from build123d import *

# Parameters (mm, degrees)
F0_W     = 11.4046361996
F0_H     = 20.0534798205
F1_DEPTH = 12.7
F3_DEPTH = 4.17264
F5_R     = 3.1549889686
F6_DEPTH = 25.4
F7_W     = 10.0605683401
F7_H     = 14.2366550863
F8_DEPTH = 7.95975


with BuildPart() as f1:
    # F0 (on Front) → F1 (new body, symmetric)
    with BuildSketch(Plane.XZ):
        Polygon((-13.2875442505, 21.1651604623), (-17.2738078982, 0), (-13.2875442505, 0), (-1.8829080509, 0), (0, 0), (0, 21.1651604623), align=None)
        with Locations((-7.5852261507, -10.0267399102)):
            Rectangle(F0_W, F0_H)
        Polygon((13.2875442505, 21.1651604623), (0, 21.1651604623), (0, 0), (1.8829080509, 0), (13.2875442505, 0), (17.2738078982, 0), align=None)
        with Locations((7.5852261507, -10.0267399102)):
            Rectangle(F0_W, F0_H)
    extrude(amount=F1_DEPTH, both=True)

    # F2 (on face) → F3 (join)
    with BuildSketch(Plane(origin=(-16.6820575494, 0, 3.1419123751), x_dir=(0, -1, 0), z_dir=(-0.982722195, 0, 0.1850867027))):
        with BuildLine():
            Line((-13.796438463, 1.4029195299), (0, 2.9041063972))
            ThreePointArc((0, 2.9041063972), (5.3533335924, 7.9779976513), (0, 13.0518889055))
            Line((0, 13.0518889055), (-7.7627915889, 8.660916239))
            Line((-7.7627915889, 8.660916239), (-19.0092052332, 5.8628071696))
            ThreePointArc((-19.0092052332, 5.8628071696), (-18.616808085, 4.3270320221), (-19.026460126, 2.7957691345))
            Line((-19.026460126, 2.7957691345), (-13.796438463, 1.4029195299))
        make_face()
        with BuildLine():
            ThreePointArc((-23.0272375047, 1.4844691614), (-20.7737198496, 1.3678224494), (-19.026460126, 2.7957691345))
            ThreePointArc((-19.026460126, 2.7957691345), (-18.616808085, 4.3270320221), (-19.0092052332, 5.8628071696))
            ThreePointArc((-19.0092052332, 5.8628071696), (-21.0317417116, 7.3939934823), (-23.5248878598, 6.9255838171))
            Line((-23.5248878598, 6.9255838171), (-23.5248878598, 5.4076067172))
            ThreePointArc((-23.5248878598, 5.4076067172), (-19.7584909862, 4.1445688112), (-23.5248878598, 2.8815309051))
            Line((-23.5248878598, 2.8815309051), (-23.0272375047, 1.4844691614))
        make_face()
    extrude(amount=F3_DEPTH)

    # F4: F1 across plane


with BuildPart() as f1_1:
    add(f1.part)
    add(f1.part.mirror(Plane.YZ))

    # F5 (on Top) → F6 (join)
    with BuildSketch(Plane.XY):
        Circle(F5_R)
    extrude(amount=F6_DEPTH)

    # F7 (on Front) → F8 (join)
    with BuildSketch(Plane.XZ):
        with Locations((5.0302841701, 30.1817078143)):
            Rectangle(F7_W, F7_H)
        with Locations((-5.0302841701, 30.1817078143)):
            Rectangle(F7_W, F7_H)
    extrude(amount=-F8_DEPTH)


solid = f1_1.part
Geometry check sheet. Reference: the model listing, model coordinates, mm. A direction names the side the tool comes from. Round coordinates to 2 decimals unless told otherwise and drop trailing zeros. Write each loop counter-clockwise with the first axis right and the second up, starting at its lowest first coordinate (ties: lowest second). Pieces come first, ordered by that corner, then holes. Notation, with made-up numbers: (15, 65) -> (29, 65) arc R18 ccw to (29, 95) -> close; hole circle Ø6 at (65, 56). An arc over 180 degrees is marked (long way). One line per item, written item: value. Start each with the question number.
(1) Draft check along X on faces 1 (the cylindrical face through (17.92, 19.76, 7.67)), 2 (the flat face through (-1.883, 0, -10)), 3 (the flat face through (-19.69, 6.08, 9.71)), 4 (the flat face through (0, -12.7, 1)). Enter one of: +X half, -X half, draft (parallel to the pull), parting line (faces both ways), or undercut.
(2) Go/stop test with flat-tipped pins: pin 1 Ø4.5 at (x, z) = (1.5, 27.5) entering from -Y; pin 2 Ø4 at (y, z) = (4, 28) entering from +X; pin 3 Ø15.5 at (x, z) = (-4.5, 29.5) entering from +Y. Record where each tip stops, or that it passes through.
(3) Cross-section at A-A, the plane z = -11. Record the cut outline in (x, y).
(4) Cross-section at C-C, the plane x = 0. Record the cut outline in (y, z), and give its area (3 significant figures).
(5) Scan lines: line 1 (X direction, y = -8.5, z = -8.5); line 2 (Z direction, x = 10, y = 6); line 3 (Y direction, x = -8, z = -1). Record each from-to range of solid material in increasing order. Write a range as [from, to].
(6) Cross-section at B-B, the plane x = -9. Record the cut outline in (y, z), and give its area (3 significant figures).
(7) Access from +Z, -Z, +X, -X, +Y, -Y to the whole of each face (thin tool, end or side, straight path). Record for faces 5 (the flat face through (15, 0, 0)), 6 (the cylindrical face through (17.34, 21, 10.78)), 7 (the cylindrical face through (-0.68, -3.08, 22.78)), 8 (the flat face through (-18.31, 6.99, 5.63)).
(8) Cross-section at D-D, the plane y = 10. Record the cut outline in (x, z), and give its area (3 significant figures).
Answer:
1. face 1: undercut
1. face 2: undercut
1. face 3: -X half
1. face 4: draft
2. pin 1: y = -3.08
2. pin 2: x = 10.06
2. pin 3: y = 7.96
3. outline: (-13.29, -12.7) -> (-1.88, -12.7) -> (-1.88, 12.7) -> (-13.29, 12.7) -> close; (1.88, -12.7) -> (13.29, -12.7) -> (13.29, 12.7) -> (1.88, 12.7) -> close
4. outline: (-12.7, 0) -> (12.7, 0) -> (12.7, 21.17) -> (3.15, 21.17) -> (3.15, 23.06) -> (7.96, 23.06) -> (7.96, 37.3) -> (0, 37.3) -> (0, 25.4) -> (-3.15, 25.4) -> (-3.15, 21.17) -> (-12.7, 21.17) -> close
4. area: 670 mm²
5. line 1: [-13.29, -1.88], [1.88, 13.29]
5. line 2: [-20.05, 21.17], [23.06, 37.3]
5. line 3: [-12.7, 12.7]
6. outline: (-12.7, -20.05) -> (12.7, -20.05) -> (12.7, 21.17) -> (-12.7, 21.17) -> close; (0, 23.06) -> (7.96, 23.06) -> (7.96, 37.3) -> (0, 37.3) -> close
6. area: 1,160 mm²
7. face 5: -Z, +X, +Y, -Y
7. face 6: +Z
7. face 7: none
7. face 8: -X, -Y
8. outline: (-20.45, 5.7) -> (-16.35, 4.93) -> (-17.27, 0) -> (-13.29, 0) -> (-13.29, -20.05) -> (-1.88, -20.05) -> (-1.88, 0) -> (1.88, 0) -> (1.88, -20.05) -> (13.29, -20.05) -> (13.29, 0) -> (17.27, 0) -> (16.35, 4.93) -> (20.45, 5.7) -> (19.28, 11.88) -> (15.18, 11.11) -> (13.29, 21.17) -> (-13.29, 21.17) -> (-15.18, 11.11) -> (-19.28, 11.88) -> close
8. area: 1,160 mm²
